Work out the finished part from the listing and answer in its coordinate system (mm). Face numbers are marked on the shaded views. Coordinates: 2 decimals unless noted, no trailing zeros. Order: outer loops, then holes, each group sorted by start corner. A loop starts at its lowest first (then second) coordinate and runs counter-clockwise, first axis right, second up. Notation, with made-up numbers: M 65.5,15 L 123.5,15 A26 ccw 123.5,43 Z; hole C 58,38.5 d8. An arc over 180 degrees is marked long. Write item = value, one per line. Start each with the question number.
Q1. Find section B-B on z = -305. Give the vertices of the cut face in (x, y), and give its area (3 significant figures).
Q2. Determine the mould class of the marked faces 1, 2 and 3 for opening direction Z: released by +Z, released by -Z, zero draft, split by the parting line, or undercut.
Q3. Find section D-D on z = -70. Give the vertices of the cut face in (x, y).
Q4. Find section C-C on y = 174.5. Give the vertices of the cut face in (x, z), and give its area (3 significant figures).
Q5. Straight lines are drawn through the part: line 1 along X through (y, z) = (11, -40); line 2 along Z through (x, y) = (11.5, 17); line 3 along X through (y, z) = (14, -294.64) (3 decimals). For each, find the intervals that lie inside material, in ascending order.
Q6. Each of these flat-tipped pins is pushed along its axis until it touches: P1, Ø1.5, axis at x = 10, z = -348.5, coming from the +Y side; P2, Ø5.5, axis at x = 12.7, y = 76.2, coming from the -Z side; P3, Ø6, axis at x = 21, z = -126.5, coming from the +Y side. Where does it stop, or does it pass through?
Q7. Find section A-A on y = 119. Give the vertices of the cut face in (x, z), and give its area (3 significant figures).
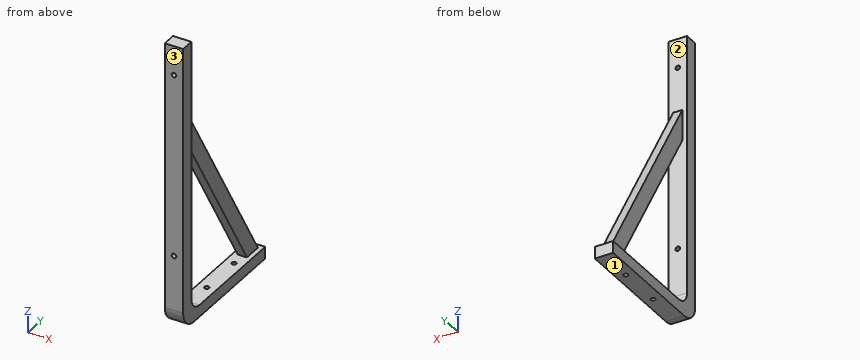
```python
from build123d import *

# Parameters (mm, degrees)
F1_DEPTH  = 25.4
F2_R      = 25.4
F3_R      = 19.05
F5_DEPTH  = 25.4
F7_DEPTH  = 6.35
F9_DEPTH  = 6.35
F10_R     = 3.175
F11_DEPTH = 25.4
F12_R     = 3.175
F13_DEPTH = 25.4


with BuildPart() as f1:
    # F0 (on Right) → F1 (new body)
    with BuildSketch(Plane.YZ):
        Polygon((19.05, 0), (0, 0), (0, -396.24), (190.5, -396.24), (190.5, -379.73), (19.05, -379.73), align=None)
    extrude(amount=F1_DEPTH)

    # F2
    f2_edges = [f1.edges().sort_by_distance(p)[0] for p in [
        (12.7, 0, -396.24),
    ]]
    fillet(f2_edges, radius=F2_R)

    # F3
    f3_edges = [f1.edges().sort_by_distance(p)[0] for p in [
        (12.7, 19.05, -379.73),
    ]]
    fillet(f3_edges, radius=F3_R)

    # F4 (on face) → F5 (join)
    with BuildSketch(Plane(origin=(0, 0, 0), x_dir=(0, -1, 0), z_dir=(-1, 0, 0))):
        Polygon((-19.05, -101.6), (-184.15, -379.73), (-158.75, -379.73), (-19.05, -144.389231), align=None)
    extrude(amount=-F5_DEPTH)

    # F6 (on face) → F7 (cut)
    with BuildSketch(Plane(origin=(0, 0, 0), x_dir=(0, -1, 0), z_dir=(-1, 0, 0))):
        Polygon((-19.05, -144.389231), (-19.05, -101.6), (-184.15, -379.73), (-158.75, -379.73), align=None)
    extrude(amount=-F7_DEPTH, mode=Mode.SUBTRACT)

    # F8 (on face) → F9 (cut)
    with BuildSketch(Plane.YZ.offset(25.4)):
        Polygon((158.75, -379.73), (184.15, -379.73), (19.05, -101.6), (19.05, -144.389231), align=None)
    extrude(amount=-F9_DEPTH, mode=Mode.SUBTRACT)

    # F10 (on face) → F11 (cut)
    with BuildSketch(Plane.XY.offset(-379.73)):
        with Locations((12.7, 76.2)):
            Circle(F10_R)
        with Locations((12.7, 139.7)):
            Circle(F10_R)
    extrude(amount=-F11_DEPTH, mode=Mode.SUBTRACT)

    # F12 (on face) → F13 (cut)
    with BuildSketch(Plane.XZ):
        with Locations((12.7, -40.64)):
            Circle(F12_R)
        with Locations((12.7, -294.64)):
            Circle(F12_R)
    extrude(amount=-F13_DEPTH, mode=Mode.SUBTRACT)


solid = f1.part
```
Findings below:
q1.outline = M 0,0 L 25.4,0 L 25.4,19.05 L 0,19.05 Z; M 6.35,114.39 L 19.05,114.39 L 19.05,139.79 L 6.35,139.79 Z
q1.area = 806 mm^2
q2.face_1 = released by -Z
q2.face_2 = undercut
q2.face_3 = zero draft
q3.outline = M 0,0 L 25.4,0 L 25.4,19.05 L 0,19.05 Z
q4.outline = M 0,-396.24 L 25.4,-396.24 L 25.4,-379.73 L 19.05,-379.73 L 19.05,-363.47 L 6.35,-363.47 L 6.35,-379.73 L 0,-379.73 Z
q4.area = 626 mm^2
q5.line_1 = 0 to 9.59, 15.81 to 25.4
q5.line_2 = -394.81 to -297.58, -291.7 to -43.58, -37.7 to 0
q5.line_3 = 0 to 9.525, 15.875 to 25.4
q6.P1 = 166.06
q6.P2 = -245.3
q6.P3 = 35.18
q7.outline = M 0,-396.24 L 25.4,-396.24 L 25.4,-379.73 L 0,-379.73 Z; M 6.35,-312.77 L 19.05,-312.77 L 19.05,-269.98 L 6.35,-269.98 Z
q7.area = 963 mm^2
